Verification items for the finished model (mm, model axes). Give positions to 0.01 mm unless a question says otherwise; leave off trailing zeros. Write each loop counter-clockwise with the first axis right and the second up, starting at its lowest first coordinate (ties: lowest second). Pieces come first, ordered by that corner, then holes. Notation, with made-up numbers: M 33,-21 L 47,-21 A28 cw 47,11 Z; hole C -21,-8.5 d7. An arc over 180 degrees is marked long. Answer as a JSON object with one key per item and string values.
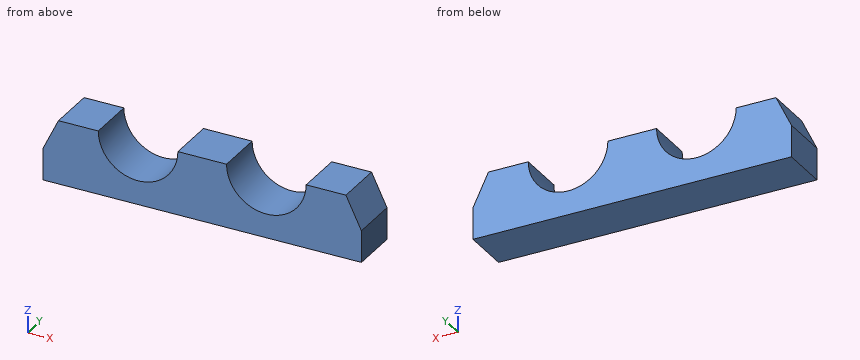
```python
from build123d import *

# Parameters (mm, degrees)
F1_DEPTH = 15


with BuildPart() as f1:
    # F0 (on Front) → F1 (new body)
    with BuildSketch(Plane.XZ):
        with BuildLine():
            Line((-19.085956, 10), (-19.085956, 0))
            Line((-19.085956, 0), (80.914044, 0))
            Line((80.914044, 0), (80.914044, 10))
            Line((80.914044, 10), (76.056394, 20))
            Line((76.056394, 20), (63.556394, 20))
            ThreePointArc((63.556394, 20), (51.056394, 7.5), (38.556394, 20))
            Line((38.556394, 20), (23.271694, 20))
            ThreePointArc((23.271694, 20), (10.771694, 7.5), (-1.728306, 20))
            Line((-1.728306, 20), (-14.228306, 20))
            Line((-14.228306, 20), (-19.085956, 10))
        make_face()
    extrude(amount=F1_DEPTH)


solid = f1.part
```
1) Section check C-C on x = 11. Record the boundary of the cut face in (y, z), and give its area (3 significant figures).
Completed:
{"outline": "M -15,0 L 0,0 L 0,7.5 L -15,7.5 Z", "area": "113 mm2"}
2) Section check D-D on x = 52.5. Record the boundary of the cut face in (y, z), and give its area (3 significant figures).
Completed:
{"outline": "M -15,0 L 0,0 L 0,7.58 L -15,7.58 Z", "area": "114 mm2"}
3) Go/stop test with flat-tipped pins: pin 1 (4 mm diameter, centred on x = 8, y = -12, fed in from +Z); pin 2 (1.5 mm diameter, centred on y = -2.5, z = 11, fed in from -X). Record where each tip stops, or that it passes through.
Completed:
{"pin 1": "stops at z = 8.45", "pin 2": "stops at x = -18.96"}
4) Section check A-A on y = -8.75. Record the boundary of the cut face in (x, z), and give its area (3 significant figures).
Completed:
{"outline": "M -19.09,0 L 80.91,0 L 80.91,10 L 76.06,20 L 63.56,20 A12.5 cw 38.56,20 L 23.27,20 A12.5 cw -1.73,20 L -14.23,20 L -19.09,10 Z", "area": "1,460 mm2"}
5) Section check B-B on z = 11. Record the boundary of the cut face in (x, y).
Completed:
{"outline": "M -18.6,-15 L 2.1,-15 L 2.1,0 L -18.6,0 Z; M 19.45,-15 L 42.38,-15 L 42.38,0 L 19.45,0 Z; M 59.73,-15 L 80.43,-15 L 80.43,0 L 59.73,0 Z"}
6) Thickness scan on L1, parallel to X at y = -14, z = 17.75; L2, parallel to X at y = -8, z = 15.75; L3, parallel to Z at x = 3.5, y = -12.5. Record the ranges inside material, lowest first.
Completed:
{"L1": "x = -15.32 to -1.52, 23.07 to 38.76, 63.35 to 77.15", "L2": "x = -16.29 to -0.98, 22.53 to 39.3, 62.81 to 78.12", "L3": "z = 0 to 9.83"}
